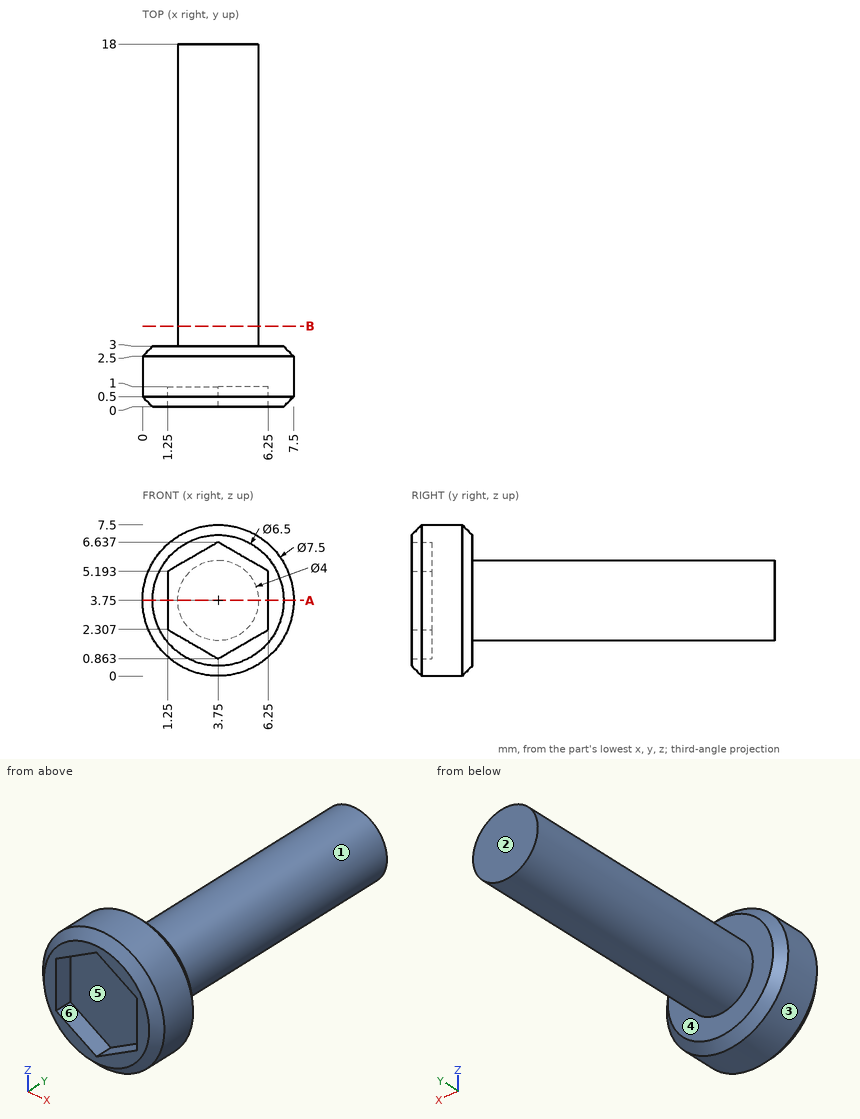
Study the drawing (mm; zero at the part's minimum x, y, z) and answer. A direction names the side the tool comes from. Round coordinates to 2 decimals unless told otherwise and drop trailing zeros. Write each loop counter-clockwise with the first axis right and the second up, starting at its lowest first coordinate (ties: lowest second). Pieces come first, ordered by that corner, then holes.
Q1. Flat-ended cylindrical pins translate along their axes: P1, Ø2, axis at x = 4, z = 2.5, coming from the -Y side; P2, Ø3, axis at x = 3.5, y = 8, coming from the -Z side. Find the tip coordinate at first contact, or state that the pin passes through.
Values:
P1: stops at y = 1
P2: stops at z = 1.75
Q2. A tool of negligible diameter and unlimited length cuts with its end or side. For the marked faces 1 and 2, from which of +Z, -Z, +X, -X, +Y, -Y can it reach the whole face along a straight path? Write none if from no direction.
Values:
face 1: +Y
face 2: +Z, -Z, +X, -X, +Y
Q3. Find section B-B on y = 4. Determine the outline of the cut face in (x, z), and give its area (3 significant figures).
Values:
outline: circle Ø4 at (3.75, 3.75)
area: 12.6 mm2
Q4. Straight lines are drawn through the part: line 1 (Y direction, x = 3.5, z = 4.75); line 2 (Y direction, x = 6.25, z = 5.25); line 3 (X direction, y = 16, z = 2.5). For each, find the intervals that lie inside material, in ascending order.
Values:
line 1: y = 1 to 18
line 2: y = 0 to 3
line 3: x = 2.19 to 5.31
Q5. The mould has two halves that part along Z. Classify the marked faces 3, 4, 5 and 6: released by +Z, released by -Z, zero draft, split by the parting line, or undercut.
Values:
face 3: split by the parting line
face 4: zero draft
face 5: undercut
face 6: undercut
Q6. Find section A-A on z = 3.75. Determine the outline of the cut face in (x, y).
Values:
outline: (0, 0.5) - (0.5, 0) - (1.25, 0) - (1.25, 1) - (6.25, 1) - (6.25, 0) - (7, 0) - (7.5, 0.5) - (7.5, 2.5) - (7, 3) - (5.75, 3) - (5.75, 18) - (1.75, 18) - (1.75, 3) - (0.5, 3) - (0, 2.5) - close
